Work out the finished part from the listing and answer in its coordinate system (mm). Give positions to 0.01 mm unless a question says otherwise; leave off trailing zeros. Write each loop counter-clockwise with the first axis right and the second up, starting at its lowest first coordinate (ties: lowest second). Pieces come first, ordered by that corner, then holes. Notation, with made-up numbers: (-14, 19.25) - (6, 19.25) arc R24 cw to (6, 50.25) - close; hole circle Ø1 at (22.25, 73). An arc over 180 degrees is marked (long way). Write item = value, one per line.
from build123d import *

# Parameters (mm, degrees)
SKETCH1_R           = 16
SKETCH1_R_2         = 4.5
SKETCH1_R_3         = 1.05
BOSS_EXTRUDE1_DEPTH = 2


with BuildPart() as part:
    # Sketch1 → Boss-Extrude1 (new body)
    with BuildSketch(Plane.XY):
        Circle(SKETCH1_R)
        Circle(SKETCH1_R_2, mode=Mode.SUBTRACT)
        with Locations((0, 8)):
            Circle(SKETCH1_R_3, mode=Mode.SUBTRACT)
        with Locations((8, 0)):
            Circle(SKETCH1_R_3, mode=Mode.SUBTRACT)
        with Locations((0, -8)):
            Circle(SKETCH1_R_3, mode=Mode.SUBTRACT)
        with Locations((-8, 0)):
            Circle(SKETCH1_R_3, mode=Mode.SUBTRACT)
    extrude(amount=BOSS_EXTRUDE1_DEPTH)


solid = part.part
1. Given pin 1 (1.3 mm diameter, centred on x = 0, y = 8, fed in from +Z); pin 2 (1 mm diameter, centred on x = -8, z = 1.5, fed in from -Y), each flat-ended and moving along its own axis, determine where each tip first touches the part or whether it passes through.
Solution:
pin_1 = through
pin_2 = -14.13
2. Find section A-A, the plane x = 0. Give the vertices of the cut face in (y, z).
Solution:
outline = (-16, 0) - (-9.05, 0) - (-9.05, 2) - (-16, 2) - close; (-6.95, 0) - (-4.5, 0) - (-4.5, 2) - (-6.95, 2) - close; (4.5, 0) - (6.95, 0) - (6.95, 2) - (4.5, 2) - close; (9.05, 0) - (16, 0) - (16, 2) - (9.05, 2) - close
3. Find section C-C, the plane x = -8.5. Give the vertices of the cut face in (y, z).
Solution:
outline = (-13.56, 0) - (-0.92, 0) - (-0.92, 2) - (-13.56, 2) - close; (0.92, 0) - (13.56, 0) - (13.56, 2) - (0.92, 2) - close
4. Straight lines are drawn through the part: line 1 (Y direction, x = 0, z = 1.65); line 2 (Y direction, x = -8, z = 0.65); line 3 (X direction, y = 1.5, z = 0.65). For each, find the intervals that lie inside material, in ascending order.
Solution:
line_1 = -16 to -9.05, -6.95 to -4.5, 4.5 to 6.95, 9.05 to 16
line_2 = -13.86 to -1.05, 1.05 to 13.86
line_3 = -15.93 to -4.24, 4.24 to 15.93
5. Find section D-D, the plane z = 0.55. Give the vertices of the cut face in (x, y), then the cut area to 3 significant figures.
Solution:
outline = circle Ø32 at (0, 0); hole circle Ø2.1 at (-8, 0); hole circle Ø9 at (0, 0); hole circle Ø2.1 at (0, -8); hole circle Ø2.1 at (0, 8); hole circle Ø2.1 at (8, 0)
area = 727 mm^2
6. For a pull along X with two mould halves and no side action, classify faces 1 (the cylindrical face through (-3.47, -15.62, 0.99)), 2 (the cylindrical face through (-9.05, 0.05, 0.99)), 3 (the flat face through (3.3, -3.3, 0)) as pulls with the +X half, pulls with the -X half, needs draft (parallel to the pull), parting line crosses it, or undercut.
Solution:
face_1 = parting line crosses it
face_2 = undercut
face_3 = needs draft
7. Find section B-B, the plane y = 3. Give the vertices of the cut face in (x, z).
Solution:
outline = (-15.72, 0) - (-3.35, 0) - (-3.35, 2) - (-15.72, 2) - close; (3.35, 0) - (15.72, 0) - (15.72, 2) - (3.35, 2) - close
